Read the model definition and answer for the solid it produces. Units are mm, in the model's axes. A direction names the side the tool comes from. Give positions to 0.01 mm unless a question says otherwise; leave off trailing zeros. Order: outer loops, then holes, each group sorted by start corner. A loop starts at its lowest first (then second) coordinate and runs counter-clockwise, first axis right, second up. Notation, with made-up numbers: (-1, 17.5) - (48, 17.5) arc R25 ccw to (48, 48.5) - close; hole circle Ø3 at (51, 27). An arc over 180 degrees is marked (long way). Write item = value, one per line.
```python
from build123d import *

# Parameters (mm, degrees)
SKETCH1_R           = 3
BOSS_EXTRUDE1_DEPTH = 3.175
FILLET1_R           = 10
SKETCH2_R           = 3
CUT_EXTRUDE1_DEPTH  = 4.175


with BuildPart() as part:
    # Sketch1 → Boss-Extrude1 (new body)
    with BuildSketch(Plane.XY):
        with BuildLine():
            Line((10, 0), (10, 79.943102917))
            Line((10, 79.943102917), (127.353979946, -8.489463967))
            ThreePointArc((127.353979946, -8.489463967), (141.358485278, -6.521259098), (139.390280409, 7.483246234))
            Line((139.390280409, 7.483246234), (-10, 120.056897083))
            Line((-10, 120.056897083), (-10, 0))
            ThreePointArc((-10, 0), (0, -10), (10, 0))
        make_face()
        Circle(SKETCH1_R, mode=Mode.SUBTRACT)
        with Locations((133.372130178, -0.503108866)):
            Circle(SKETCH1_R, mode=Mode.SUBTRACT)
    extrude(amount=BOSS_EXTRUDE1_DEPTH)

    # Fillet1
    fillet1_edges = [part.edges().sort_by_distance(p)[0] for p in [
        (-10, 120.056897083, 1.5875),
        (10, 79.943102917, 1.5875),
    ]]
    fillet(fillet1_edges, radius=FILLET1_R)

    # Sketch2 → Cut-Extrude1 (cut, through all)
    with BuildSketch(Plane.XY.offset(3.175)):
        with Locations((0, 80)):
            Circle(SKETCH2_R)
    extrude(amount=-CUT_EXTRUDE1_DEPTH, mode=Mode.SUBTRACT)


solid = part.part
```
1. For faces 4 (the face through (75.977, 30.226, 1.565)), 5 (the face through (141.22, -6.7, 1.57)), determine the directions among +Z, -Z, +X, -X, +Y, -Y from which every point of the face is accessible in a straight line to the end or side of a thin tool.
Recorded:
face_4 = +Z, -Z, -Y
face_5 = +Z, -Z
2. Determine the mould class of faces 1 (the face through (73.64, 57.03, 1.57)), 2 (the face through (-0.65, 77.07, 1.61)), 3 (the face through (44, 63, 3.175)) for opening direction Y: +Y half, -Y half, draft (parallel to the pull), parting line (faces both ways), or undercut.
Recorded:
face_1 = +Y half
face_2 = undercut
face_3 = draft
3. Section A-A (x = 0) is taken. Determine the outline of the cut face in (y, z) (3 decimals).
Recorded:
outline = (-10, 0) - (-3, 0) - (-3, 3.175) - (-10, 3.175) - close; (3, 0) - (77, 0) - (77, 3.175) - (3, 3.175) - close; (83, 0) - (110, 0) - (110, 3.175) - (83, 3.175) - close
4. Flat-ended cylindrical pins translate along their axes: pin 1 (3.5 mm diameter, centred on x = 133.37, y = -0.5, fed in from +Z); pin 2 (1 mm diameter, centred on x = 89, z = 1, fed in from -Y); pin 3 (1 mm diameter, centred on y = 33, z = 1, fed in from +X). Find the tip coordinate at first contact, or state that the pin passes through.
Recorded:
pin_1 = through
pin_2 = 20.04
pin_3 = 106.19
5. Section B-B (y = 80) is taken. Determine the outline of the cut face in (x, z) (3 decimals).
Recorded:
outline = (-10, 0) - (-3, 0) - (-3, 3.175) - (-10, 3.175) - close; (3, 0) - (43.157, 0) - (43.157, 3.175) - (3, 3.175) - close
6. Straight lines are drawn through the part: L1, parallel to Y at x = 0, z = 2.15; L2, parallel to X at y = 0.5, z = 1.4; L3, parallel to X at y = 46.5, z = 3.05. For each, find the intervals that lie inside material, in ascending order. Write a range as [from, to].
Recorded:
L1 = [-10, -3], [3, 77], [83, 110]
L2 = [-10, -2.96], [2.96, 10], [115.42, 130.54], [136.2, 143.32]
L3 = [-10, 10], [54.38, 87.61]
7. Section C-C (z = 2.1) is taken. Determine the outline of the cut face in (x, y).
Recorded:
outline = (-10, 0) arc R10 ccw to (10, 0) - (10, 59.89) arc R10 cw to (26.02, 67.87) - (127.35, -8.49) arc R10 ccw to (139.39, 7.48) - (6.02, 107.99) arc R10 ccw to (-10, 100) - close; hole circle Ø6 at (0, 0); hole circle Ø6 at (0, 80); hole circle Ø6 at (133.37, -0.5)
8. Section D-D (y = 49) is taken. Determine the outline of the cut face in (x, z) (3 decimals), and give its area (3 significant figures).
Recorded:
outline = (-10, 0) - (10, 0) - (10, 3.175) - (-10, 3.175) - close; (51.063, 0) - (84.296, 0) - (84.296, 3.175) - (51.063, 3.175) - close
area = 169 mm^2
